from build123d import *

# Parameters (mm, degrees)
SKETCH2_R           = 7.5
SKETCH2_R_2         = 6
EXTRUDE8_DEPTH      = 11
SKETCH2_14_W        = 23
SKETCH2_14_H        = 23
SKETCH2_14_R        = 7.5
SKETCH2_14_R_2      = 1.5
EXTRUDE9_DEPTH      = 11
EXTRUDE9_DEPTH_BACK = 5


with BuildPart() as part:
    # Sketch2 → Extrude8 (new body)
    with BuildSketch(Plane.XY):
        Circle(SKETCH2_R)
        Circle(SKETCH2_R_2, mode=Mode.SUBTRACT)
    extrude(amount=EXTRUDE8_DEPTH)

    # Sketch2<14> → Extrude9 (add, two sides)
    with BuildSketch(Plane.XY) as extrude9_sk:
        Rectangle(SKETCH2_14_W, SKETCH2_14_H)
        Circle(SKETCH2_14_R, mode=Mode.SUBTRACT)
        with Locations((8.485281374, 8.485281374)):
            Circle(SKETCH2_14_R_2, mode=Mode.SUBTRACT)
        with Locations((8.485281374, -8.485281374)):
            Circle(SKETCH2_14_R_2, mode=Mode.SUBTRACT)
        with Locations((-8.485281374, -8.485281374)):
            Circle(SKETCH2_14_R_2, mode=Mode.SUBTRACT)
        with Locations((-8.485281374, 8.485281374)):
            Circle(SKETCH2_14_R_2, mode=Mode.SUBTRACT)
    extrude(amount=EXTRUDE9_DEPTH)
    extrude(extrude9_sk.sketch, amount=-EXTRUDE9_DEPTH_BACK)


solid = part.part
Input: part model. Units: mm. Frame: model coordinates. A direction names the side the tool comes from. Round coordinates to 2 decimals unless told otherwise and drop trailing zeros. Order: outer loops, then holes, each group sorted by start corner. A loop starts at its lowest first (then second) coordinate and runs counter-clockwise, first axis right, second up.
1. Mould query, pull axis Y, two halves, no side actions, for faces 1 (the face through (0, 11.5, 3)), 2 (the face through (9.29, 9.75, 2.89)), 3 (the face through (11.5, 0, 3)). Classes: released by +Y, released by -Y, zero draft, split by the parting line, or undercut.
The answers:
face 1: released by +Y
face 2: undercut
face 3: zero draft
2. Material intervals for line 1 (Y direction, x = 8.5, z = 5); line 2 (Y direction, x = 9.5, z = -2), sorted ascending.
The answers:
line 1: y = -11.5 to -9.99, -6.99 to 6.99, 9.99 to 11.5
line 2: y = -11.5 to -9.59, -7.38 to 7.38, 9.59 to 11.5
3. Set-up query: faces 4 (the face through (0, -11.5, 3)), 5 (the face through (-7.493, 0.33, -2.465)). Return all of +Z, -Z, +X, -X, +Y, -Y with unobstructed straight access to the full face (end or side cutting, diameter ignored); none if empty.
The answers:
face 4: +Z, -Z, +X, -X, -Y
face 5: -Z
4. Cut plane D-D, the plane z = -3. Output: boundary loops of the cut face in (x, y).
The answers:
outline: (-11.5, -11.5) - (11.5, -11.5) - (11.5, 11.5) - (-11.5, 11.5) - close; hole circle Ø3 at (-8.49, -8.49); hole circle Ø3 at (-8.49, 8.49); hole circle Ø15 at (0, 0); hole circle Ø3 at (8.49, -8.49); hole circle Ø3 at (8.49, 8.49)
5. Pin query (flat end, axial travel): P1, Ø12, axis at x = 2.5, y = 2.5, coming from the -Z side; P2, Ø8, axis at x = -2.5, y = 1, coming from the -Z side. Return the tip coordinate at first contact, or that it passes through.
The answers:
P1: stops at z = -5
P2: stops at z = 0
6. Cut plane A-A, the plane x = 0. Output: boundary loops of the cut face in (y, z).
The answers:
outline: (-11.5, -5) - (-7.5, -5) - (-7.5, 0) - (-6, 0) - (-6, 11) - (-11.5, 11) - close; (6, 0) - (7.5, 0) - (7.5, -5) - (11.5, -5) - (11.5, 11) - (6, 11) - close
7. Cut plane C-C, the plane z = 1. Output: boundary loops of the cut face in (x, y), then the cut area to 3 significant figures.
The answers:
outline: (-11.5, -11.5) - (11.5, -11.5) - (11.5, 11.5) - (-11.5, 11.5) - close; hole circle Ø3 at (-8.49, -8.49); hole circle Ø3 at (-8.49, 8.49); hole circle Ø12 at (0, 0); hole circle Ø3 at (8.49, -8.49); hole circle Ø3 at (8.49, 8.49)
area: 388 mm2
